Here's how the part is built. I have some questions about the finished solid (model axes, mm). Face numbers are marked on the shaded views. A direction names the side the tool comes from. Round coordinates to 2 decimals unless told otherwise and drop trailing zeros. Write each loop counter-clockwise with the first axis right and the second up, starting at its lowest first coordinate (ties: lowest second). Pieces come first, ordered by that corner, then holes. Notation, with made-up numbers: (51, 55.5) - (81, 55.5) arc R19 cw to (81, 73.5) - close; hole circle Ø1 at (37.5, 44.5). An arc over 180 degrees is marked (long way). One line per item, written item: value. Start each with the question number.
Item 1: For the marked faces 5 and 6, which set-ups out of +Z, -Z, +X, -X, +Y, -Y let a thin tool reach every point of the face, with its end or its side?
Item 2: Thinking about a two-plate mould opening in X: for the marked faces 1, 2, 3 and 4, which applies, released by +X, released by -X, zero draft, split by the parting line, or undercut?
Item 3: Imagine slicing it at A-A, the plane z = 8.5. Please give me the cut outline in (x, y).
Item 4: Imagine slicing it at B-B, the plane y = 1.5. Count the separate pieces of the cut face and the enclosed holes in it, then the cut area to 3 significant figures.
Item 5: If I drill on line 1 (X direction, y = 2, z = -2.5); line 2 (X direction, y = 4.75, z = 0.75); line 3 (Z direction, x = 5.75, y = 3.5), over which ranges is the centre line in solid material (lowest first)?
Item 6: For P1, Ø8, axis at x = -2, y = 9, coming from the +Z side; P2, Ø3, axis at x = 0.5, z = 0.5, coming from the +Y side; P3, Ø1.1, axis at y = 2.5, z = 4, coming from the +X side, each with a flat end and sliding along its axis, tell me the tip position at first contact or that it passes through.
```python
from build123d import *

# Parameters (mm, degrees)
SKETCH1_W                = 12
SKETCH1_H                = 1.6
BOSS_EXTRUDE1_DEPTH      = 15
BOSS_EXTRUDE1_TAPER      = -7
SHELL1_T                 = -0.5
SKETCH6_W                = 3.4
SKETCH6_H                = 20
BOSS_EXTRUDE2_DEPTH      = 3.5
BOSS_EXTRUDE2_2_DEPTH    = 3.5
CUT_EXTRUDE11_DEPTH      = 10
CUT_EXTRUDE11_DEPTH_BACK = 10
SKETCH11_RX              = 4.5
SKETCH11_RY              = 1.5
CUT_EXTRUDE12_DEPTH      = 10
BOSS_EXTRUDE3_DEPTH      = 0.5
SKETCH30_W               = 3.2
SKETCH30_H               = 1.6
BOSS_EXTRUDE6_DEPTH      = 9
BOSS_EXTRUDE6_TAPER      = -6
SKETCH31_R               = 1.504583892
BOSS_EXTRUDE7_DEPTH      = 2
BOSS_EXTRUDE7_TAPER      = 10
SKETCH32_R               = 0.64546473
CUT_EXTRUDE13_DEPTH      = 4


with BuildPart() as part:
    # Sketch1 → Boss-Extrude1 (new body)
    with BuildSketch(Plane(origin=(0, 0, 0), x_dir=(1, 0, 0), z_dir=(0, 1, 0))):
        Rectangle(SKETCH1_W, SKETCH1_H)
    extrude(amount=BOSS_EXTRUDE1_DEPTH, taper=BOSS_EXTRUDE1_TAPER)

    # Shell1
    shell1_openings = [part.faces().sort_by_distance(p)[0] for p in [
        (0, 15, 0),
    ]]
    offset(amount=SHELL1_T, openings=shell1_openings, kind=Kind.INTERSECTION)

    # Sketch11 → Cut-Extrude11 (cut, two sides: drawn at the far end of the back side and taken through both)
    with BuildSketch(Plane.XY.offset(-CUT_EXTRUDE11_DEPTH_BACK)):
        with Locations((0, 15)):
            Ellipse(SKETCH11_RX, SKETCH11_RY)
    extrude(amount=CUT_EXTRUDE11_DEPTH + CUT_EXTRUDE11_DEPTH_BACK, mode=Mode.SUBTRACT)

    # Sketch18 → Cut-Extrude12 (cut, symmetric)
    with BuildSketch(Plane.XY):
        Polygon((-2.966549011, 13.872092056), (-7.173702506, 9.559039808), (-8.984967274, 15.813419698), (-2.966549011, 15.813419698), align=None)
    cut_extrude12 = extrude(amount=CUT_EXTRUDE12_DEPTH, both=True, mode=Mode.SUBTRACT)

    # Sketch19 → Boss-Extrude3 (add)
    with BuildSketch(Plane(origin=(-8.45404379, 8.246470904, 0), x_dir=(0, 0, 1), z_dir=(-0.7158402135047951, 0.6982641253346826, 0))):
        Polygon((1.973702506, 1.833605992), (2.503278732, 7.858766589), (-2.503278732, 7.858766589), (-1.973702506, 1.833605992), align=None)
    boss_extrude3 = extrude(amount=-BOSS_EXTRUDE3_DEPTH)

    # Mirror3: Boss-Extrude3 across plane
    add(boss_extrude3.mirror(Plane(origin=(0, 0, 0), x_dir=(0, 0, 1), z_dir=(1, 0, 0))))



with BuildPart() as body_2:
    # Sketch6 → Boss-Extrude2 (new body)
    with BuildSketch(Plane.XZ):
        with Locations((-3.3, 0)):
            Rectangle(SKETCH6_W, SKETCH6_H)
    extrude(amount=-BOSS_EXTRUDE2_DEPTH)


with BuildPart() as body_3:
    # Sketch6 → Boss-Extrude2 2 (new body)
    with BuildSketch(Plane.XZ):
        with Locations((3.3, 0)):
            Rectangle(SKETCH6_W, SKETCH6_H)
    extrude(amount=-BOSS_EXTRUDE2_2_DEPTH)


with BuildPart() as part_1:
    add(part.part)

    add(body_2.part)  # Boss-Extrude6 merges body 2

    add(body_3.part)  # Boss-Extrude6 merges body 3
    # Sketch30 → Boss-Extrude6 (add)
    with BuildSketch(Plane.XZ):
        Rectangle(SKETCH30_W, SKETCH30_H)
    extrude(amount=-BOSS_EXTRUDE6_DEPTH, taper=BOSS_EXTRUDE6_TAPER)

    # Mirror7: Cut-Extrude12 across plane
    add(cut_extrude12.mirror(Plane(origin=(0, 0, 0), x_dir=(0, 0, 1), z_dir=(1, 0, 0))), mode=Mode.SUBTRACT)

    # Sketch31 → Boss-Extrude7 (add)
    with BuildSketch(Plane(origin=(5.910887179, -0.725765687, 0), x_dir=(0, 0, -1), z_dir=(0.992546151641322, -0.12186934340514774, 0))):
        with Locations((0, 7.63302961)):
            Circle(SKETCH31_R)
    boss_extrude7 = extrude(amount=BOSS_EXTRUDE7_DEPTH, taper=BOSS_EXTRUDE7_TAPER)

    # Mirror8: Boss-Extrude7 across plane
    add(boss_extrude7.mirror(Plane(origin=(0, 0, 0), x_dir=(0, 0, 1), z_dir=(1, 0, 0))))

    # Sketch32 → Cut-Extrude13 (cut)
    with BuildSketch(Plane(origin=(7.895979482, -0.969504374, 0), x_dir=(0, 0, -1), z_dir=(0.992546151641322, -0.12186934340514774, 0))):
        with Locations(Location((0, 7.63302961, 0), (0, 0, 90))):
            Circle(SKETCH32_R)
    cut_extrude13 = extrude(amount=-CUT_EXTRUDE13_DEPTH, mode=Mode.SUBTRACT)

    # Mirror9: Cut-Extrude13 across plane
    add(cut_extrude13.mirror(Plane(origin=(0, 0, 0), x_dir=(0, 0, 1), z_dir=(1, 0, 0))), mode=Mode.SUBTRACT)


solid = part_1.part
```
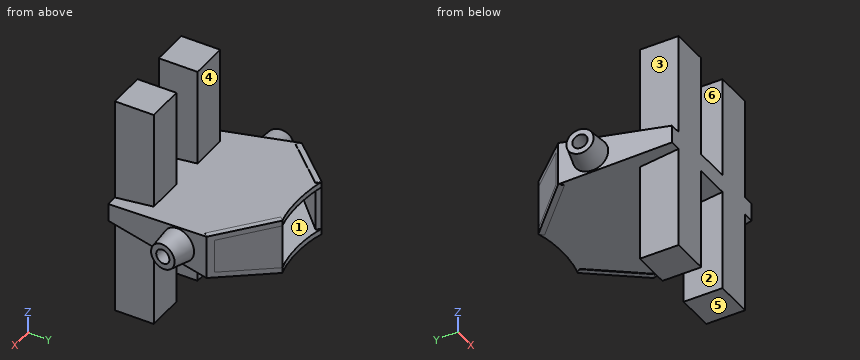
Values follow:
1. face 5: -Z, +X, -X, +Y, -Y
1. face 6: +Z, -Y
2. face 1: undercut
2. face 2: undercut
2. face 3: released by -X
2. face 4: zero draft
3. outline: (-5, 0) - (-1.6, 0) - (-1.6, 3.5) - (-5, 3.5) - close; (1.6, 0) - (5, 0) - (5, 3.5) - (1.6, 3.5) - close
4. separate pieces: 1
4. enclosed holes: 2
4. area: 146 mm^2
5. line 1: x = -5 to -1.6, 1.6 to 5
5. line 2: x = -6.58 to -6.08, -2.1 to 2.1, 6.08 to 6.58
5. line 3: z = -1.23 to -0.73, 0.73 to 1.23
6. P1: stops at z = 2.41
6. P2: stops at y = 13.53
6. P3: stops at x = 5
